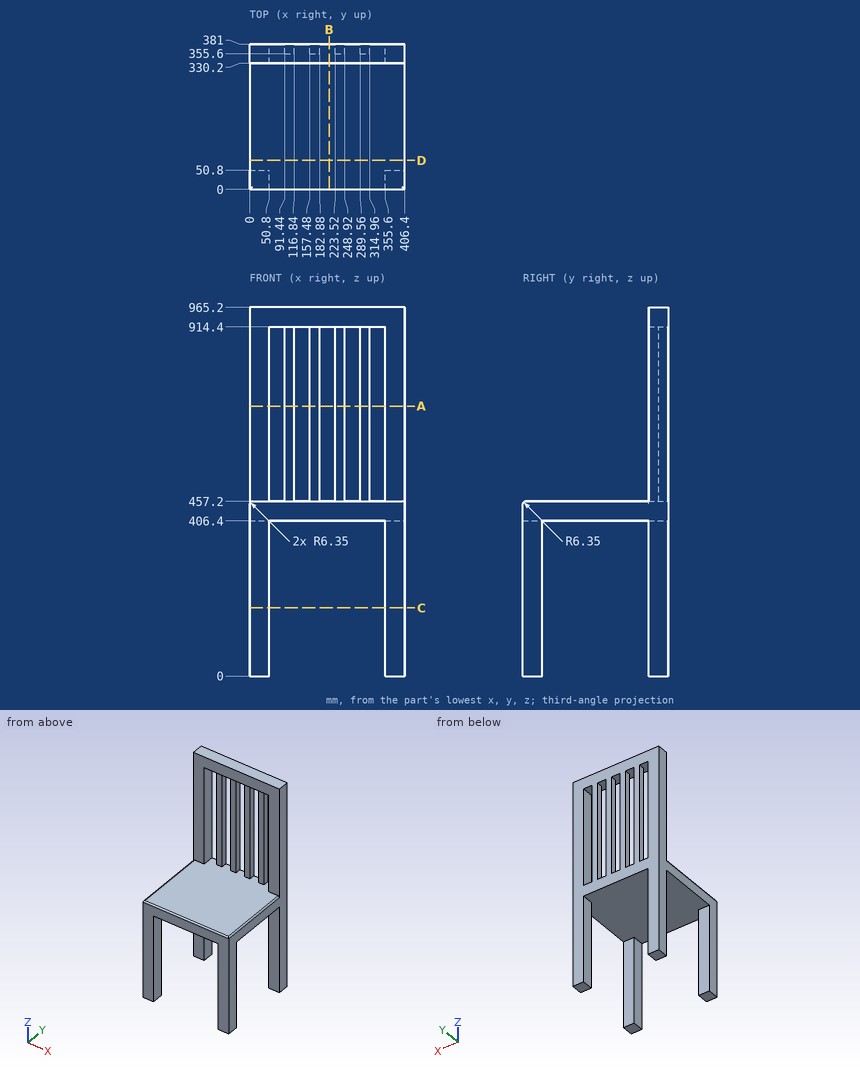
Could you check a few things on this drawing? It's one solid part, dimensions in mm from its lowest x, y, z. Give positions to 0.01 mm unless a question says otherwise; leave off trailing zeros. Order: outer loops, then holes, each group sorted by start corner. A loop starts at its lowest first (then second) coordinate and runs counter-clockwise, first axis right, second up. Notation, with made-up numbers: (59.25, 61.25) -> (76.25, 61.25) arc R30 cw to (76.25, 89.25) -> close; hole circle Ø5 at (50, -13). An arc over 180 degrees is marked (long way). Use CSV: the item, a comma, the result in double quotes. Start each with the question number.
Item 1: Suppose I cut it at A-A (z = 707). List the corners of the cut face in (x, y) for me, and give its area (3 significant figures).
Item 2: I'm going to push flat-ended pins straight in: P1, Ø20.5, axis at x = 296.5, z = 578, coming from the -Y side; P2, Ø12, axis at x = 138, z = 402.5, coming from the -Y side; P3, Ø10, axis at x = 186, y = 260, coming from the -Z side. Where does each tip first touch, or does it pass through?
Item 3: Suppose I cut it at B-B (x = 208). List the corners of the cut face in (y, z) for me.
Item 4: If I drill on probe 1 along X at (y, z) = (361.5, 879); probe 2 along X at (y, z) = (38.5, 389.5); probe 3 along Z at (x, y) = (56, 362), over which ranges is the centre line in solid material (lowest first)? Write a range as [from, to].
Item 5: Suppose I cut it at D-D (y = 76). List the corners of the cut face in (x, z) for me, and give its area (3 significant figures).
Item 6: Suppose I cut it at C-C (z = 178.5). List the corners of the cut face in (x, y) for me, and give its area (3 significant figures).
Answer block:
1,outline,"(0, 330.2) -> (50.8, 330.2) -> (50.8, 381) -> (0, 381) -> close; (91.44, 355.6) -> (116.84, 355.6) -> (116.84, 381) -> (91.44, 381) -> close; (157.48, 355.6) -> (182.88, 355.6) -> (182.88, 381) -> (157.48, 381) -> close; (223.52, 355.6) -> (248.92, 355.6) -> (248.92, 381) -> (223.52, 381) -> close; (289.56, 355.6) -> (314.96, 355.6) -> (314.96, 381) -> (289.56, 381) -> close; (355.6, 330.2) -> (406.4, 330.2) -> (406.4, 381) -> (355.6, 381) -> close"
1,area,"7,740 mm^2"
2,P1,"stops at y = 355.6"
2,P2,"stops at y = 0"
2,P3,"stops at z = 406.4"
3,outline,"(0, 406.4) -> (381, 406.4) -> (381, 457.2) -> (6.35, 457.2) arc R6.35 ccw to (0, 450.85) -> close; (330.2, 914.4) -> (381, 914.4) -> (381, 965.2) -> (330.2, 965.2) -> close"
4,probe 1,"x = [0, 50.8], [91.44, 116.84], [157.48, 182.88], [223.52, 248.92], [289.56, 314.96], [355.6, 406.4]"
4,probe 2,"x = [0, 50.8], [355.6, 406.4]"
4,probe 3,"z = [406.4, 457.2], [914.4, 965.2]"
5,outline,"(0, 406.4) -> (406.4, 406.4) -> (406.4, 450.85) arc R6.35 ccw to (400.05, 457.2) -> (6.35, 457.2) arc R6.35 ccw to (0, 450.85) -> close"
5,area,"20,600 mm^2"
6,outline,"(0, 0) -> (50.8, 0) -> (50.8, 50.8) -> (0, 50.8) -> close; (0, 330.2) -> (50.8, 330.2) -> (50.8, 381) -> (0, 381) -> close; (355.6, 0) -> (406.4, 0) -> (406.4, 50.8) -> (355.6, 50.8) -> close; (355.6, 330.2) -> (406.4, 330.2) -> (406.4, 381) -> (355.6, 381) -> close"
6,area,"10,300 mm^2"
